Part model, mm, in its own coordinate system. Face numbers are marked on the shaded views. A direction names the side the tool comes from. Round coordinates to 2 decimals unless told otherwise and drop trailing zeros. Write each loop counter-clockwise with the first axis right and the second up, starting at its lowest first coordinate (ties: lowest second). Pieces come first, ordered by that corner, then holes. Notation, with made-up numbers: (68.25, 15) -> (112.25, 15) arc R12 ccw to (112.25, 35) -> close; hole circle Ø10 at (46, 29.5). An arc over 180 degrees is marked (long way). Return JSON: item names as keys, results as strings. Group by question number.
(1) Saw through at B-B (x = 7). List the corners of the cut face in (y, z).
(2) Mould opens along X. For the marked faces 3, 4 and 5 say: +X half, -X half, draft (parallel to the pull), parting line (faces both ways), or undercut.
(3) Saw through at C-C (y = -13). List the corners of the cut face in (x, z), plus the area to 3 significant figures.
(4) Tool access for the marked faces 1 and 2: list every direction of +Z, -Z, +X, -X, +Y, -Y with a clear straight run to the whole face (end or side of a thin tool).
(5) Drill centre lines: L1, parallel to X at y = -1, z = -15; L2, parallel to X at y = 15, z = -42; L3, parallel to Z at x = -54, y = -0.5. Where is each one in solid material? Low to high. Write a range as from..to.
(6) Drop flat-ended pins along their axis: pin 1 Ø6.5 at (x, z) = (-27.5, 6) entering from +Y; pin 2 Ø5 at (x, y) = (-4, -23.5) entering from -Z; pin 3 Ø2 at (x, z) = (-16.5, -70) entering from +Y. Give the stop position or say it passes through.
(7) Saw through at A-A (z = -17). List the corners of the cut face in (x, y), plus the area to 3 significant figures.
(8) Saw through at D-D (z = 65.5). List the corners of the cut face in (x, y), plus the area to 3 significant figures.
from build123d import *

# Parameters (mm, degrees)
F0_W     = 165.1
F0_H     = 38.1
F1_DEPTH = 12.7
F2_R     = 25.4
F3_DEPTH = 101.6
F5_DEPTH = 101.6


with BuildPart() as f1:
    # F0 (on Top) → F1 (new body)
    with BuildSketch(Plane.XY):
        Rectangle(F0_W, F0_H)
    extrude(amount=F1_DEPTH)

    # F2 (on face) → F3 (join)
    with BuildSketch(Plane.XY.offset(12.7)):
        Circle(F2_R)
    extrude(amount=F3_DEPTH)

    # F4 (on face) → F5 (join)
    with BuildSketch(Plane(origin=(0, 0, 0), x_dir=(1, 0, 0), z_dir=(0, 0, -1))):
        with BuildLine():
            ThreePointArc((0, -19.05), (13.470384, -13.470384), (19.05, 0))
            ThreePointArc((19.05, 0), (13.470384, 13.470384), (0, 19.05))
            ThreePointArc((0, 19.05), (-19.05, 0), (0, -19.05))
        make_face()
        with BuildLine():
            ThreePointArc((82.55, 0), (76.970384, 13.470384), (63.5, 19.05))
            ThreePointArc((63.5, 19.05), (44.45, 0), (63.5, -19.05))
            ThreePointArc((63.5, -19.05), (76.970384, -13.470384), (82.55, 0))
        make_face()
        with BuildLine():
            ThreePointArc((-44.45, 0), (-50.029616, 13.470384), (-63.5, 19.05))
            ThreePointArc((-63.5, 19.05), (-76.970384, 13.470384), (-82.55, 0))
            ThreePointArc((-82.55, 0), (-76.970384, -13.470384), (-63.5, -19.05))
            ThreePointArc((-63.5, -19.05), (-50.029616, -13.470384), (-44.45, 0))
        make_face()
    extrude(amount=F5_DEPTH)


solid = f1.part
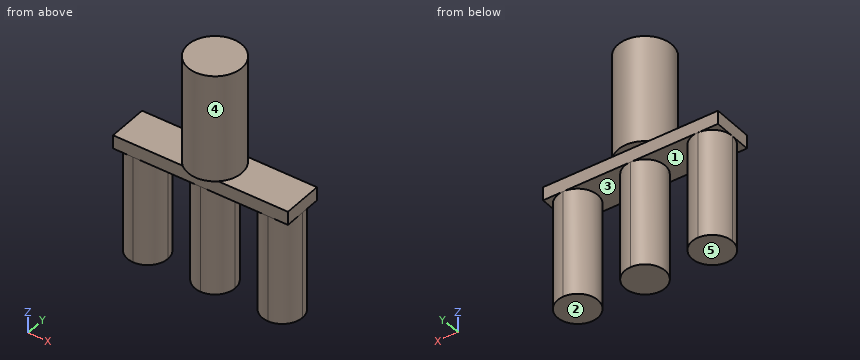
Computed values:
{
 "1": {"outline": "(-24.42, 12.7) -> (-19.05, 12.7) -> (-19.05, 0) -> (-17.72, 0) -> (-17.72, -101.6) -> (17.72, -101.6) -> (17.72, 0) -> (19.05, 0) -> (19.05, 12.7) -> (24.42, 12.7) -> (24.42, 114.3) -> (-24.42, 114.3) -> close"},
 "2": {"face 3": "undercut", "face 4": "parting line", "face 5": "draft"},
 "3": {"outline": "(-82.55, 0) -> (-77.42, 0) -> (-77.42, -101.6) -> (-49.58, -101.6) -> (-49.58, 0) -> (-13.92, 0) -> (-13.92, -101.6) -> (13.92, -101.6) -> (13.92, 0) -> (49.58, 0) -> (49.58, -101.6) -> (77.42, -101.6) -> (77.42, 0) -> (82.55, 0) -> (82.55, 12.7) -> (21.82, 12.7) -> (21.82, 114.3) -> (-21.82, 114.3) -> (-21.82, 12.7) -> (-82.55, 12.7) -> close", "area": "15,000 mm2"},
 "4": {"face 1": "-Z", "face 2": "-Z, +X, -X, +Y, -Y"},
 "5": {"L1": "-82.52..-44.48, -19.02..19.02, 44.48..82.52", "L2": "-75.24..-51.76, -11.74..11.74, 51.76..75.24", "L3": "-101.6..12.7"},
 "6": {"pin 1": "y = 19.05", "pin 2": "z = 12.7", "pin 3": "y = 11.07"},
 "7": {"outline": "(-82.55, 0) arc R19.05 ccw to (-63.5, -19.05) arc R19.05 ccw to (-44.45, 0) arc R19.05 ccw to (-63.5, 19.05) arc R19.05 ccw to start; (0, -19.05) arc R19.05 ccw to (19.05, 0) arc R19.05 ccw (long way) to start; (63.5, -19.05) arc R19.05 ccw to (82.55, 0) arc R19.05 ccw (long way) to start", "area": "3,420 mm2"},
 "8": {"outline": "circle Ø50.8 at (0, 0)", "area": "2,030 mm2"}
}
